Geometry check sheet. Reference: drawing and pictorial views, mm from the part's lowest x, y, z. Coordinates: 2 decimals unless noted, no trailing zeros. Loops run counter-clockwise (first coordinate to the right, second up) from the corner with the lowest first, then second, coordinate; pieces in that order, holes last. Notation, with made-up numbers: (-11, -19) -> (29, -19) arc R23 cw to (29, -2) -> close; hole circle Ø7 at (64, 15.5). An arc over 180 degrees is marked (long way). Answer as a JSON object with one key per item and string values. Group by question number.
Q1. Scan lines: L1, parallel to Y at x = 2.5, z = 2.5; L2, parallel to X at y = 4.25, z = 3.4; L3, parallel to X at y = 1.65, z = 2.75. Record each from-to range of solid material in increasing order.
Q2. Cross-section at D-D on z = 1.05. Record the boundary of the cut face in (x, y), and give its area (3 significant figures).
Q3. Cross-section at A-A on x = 2.5. Record the boundary of the cut face in (y, z), and give its area (3 significant figures).
Q4. Cross-section at B-B on y = 2.5. Record the boundary of the cut face in (x, z), and give its area (3 significant figures).
Q5. Release check for a two-part mould opening along X. For the marked faces 1, 2 and 3 record: released by +X, released by -X, zero draft, split by the parting line, or undercut.
Q6. Gauge pin test, flat ends, axial feed: pin 1 Ø1.5 at (y, z) = (2.5, 1.5) entering from +X; pin 2 Ø3 at (y, z) = (2.5, 3) entering from +X. Record the tip position at first contact, or that the pin passes through.
Q7. Cross-section at C-C on z = 3.35. Record the boundary of the cut face in (x, y), and give its area (3 significant figures).
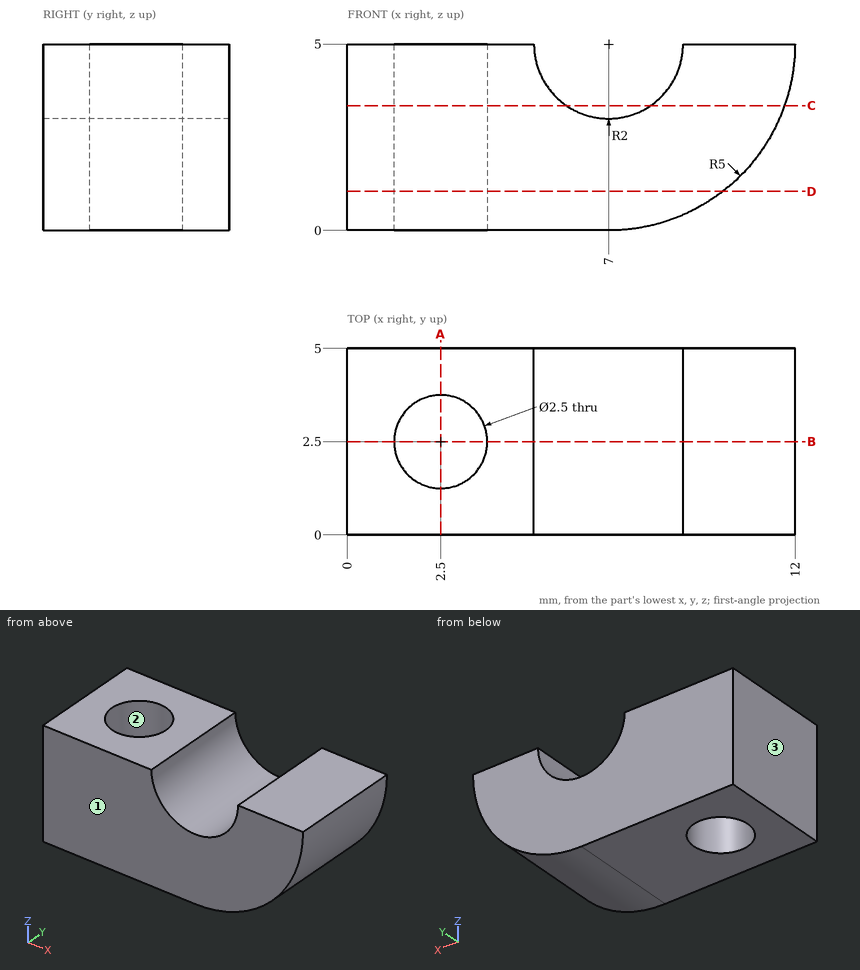
Computed values:
{
 "1": {"L1": "y = 0 to 1.25, 3.75 to 5", "L2": "x = 0 to 5.8, 8.2 to 11.74", "L3": "x = 0 to 1.58, 3.42 to 11.47"},
 "2": {"outline": "(0, 0) -> (10.07, 0) -> (10.07, 5) -> (0, 5) -> close; hole circle Ø2.5 at (2.5, 2.5)", "area": "45.4 mm²"},
 "3": {"outline": "(0, 0) -> (1.25, 0) -> (1.25, 5) -> (0, 5) -> close; (3.75, 0) -> (5, 0) -> (5, 5) -> (3.75, 5) -> close", "area": "12.5 mm²"},
 "4": {"outline": "(0, 0) -> (1.25, 0) -> (1.25, 5) -> (0, 5) -> close; (3.75, 0) -> (7, 0) arc R5 ccw to (12, 5) -> (9, 5) arc R2 cw to (5, 5) -> (3.75, 5) -> close", "area": "35.9 mm²"},
 "5": {"face 1": "zero draft", "face 2": "undercut", "face 3": "released by -X"},
 "6": {"pin 1": "stops at x = 11.18", "pin 2": "stops at x = 11.97"},
 "7": {"outline": "(0, 0) -> (5.87, 0) -> (5.87, 5) -> (0, 5) -> close; (8.13, 0) -> (11.72, 0) -> (11.72, 5) -> (8.13, 5) -> close; hole circle Ø2.5 at (2.5, 2.5)", "area": "42.4 mm²"}
}
